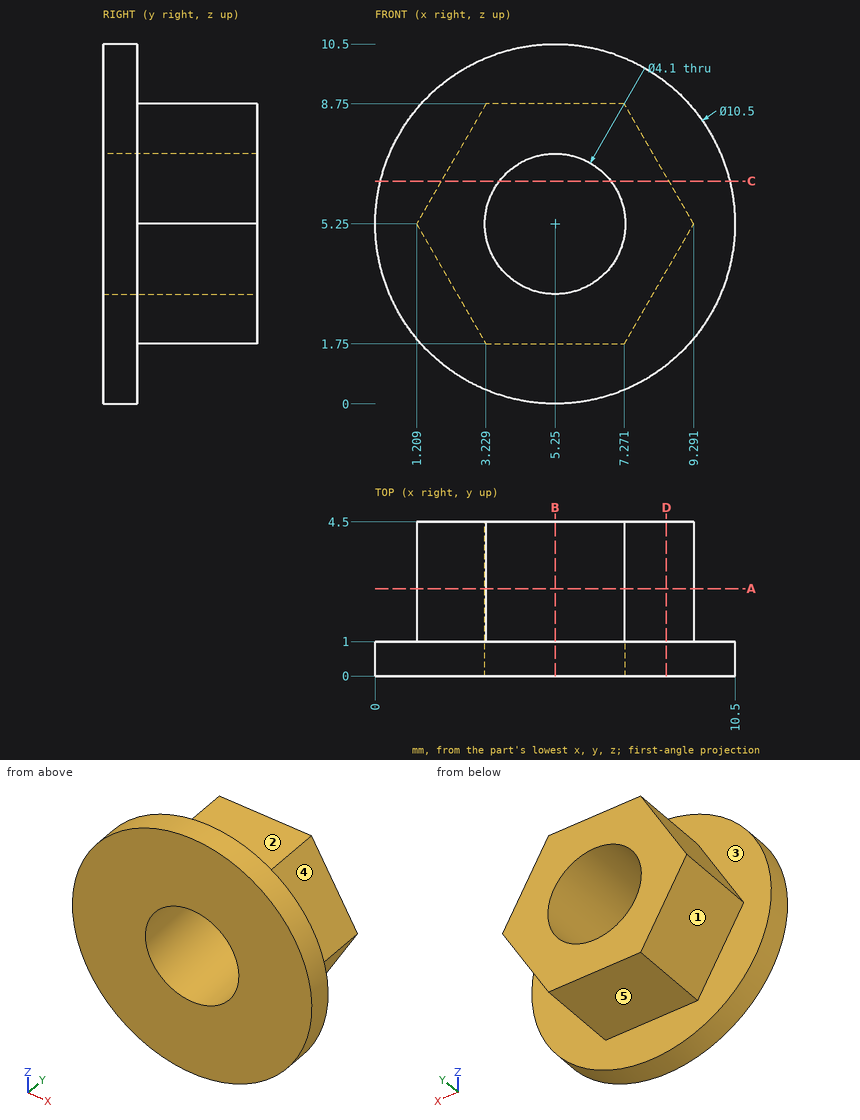
Here's the drawing with two shaded views (mm, measured from the low corner). I have some questions. A direction names the side the tool comes from. Give positions to 0.01 mm unless a question says otherwise; leave off trailing zeros. Loops run counter-clockwise (first coordinate to the right, second up) from the corner with the lowest first, then second, coordinate; pieces in that order, holes last. Notation, with made-up numbers: M 67,43 L 78,43 A12 ccw 78,58 Z; hole C 83.5,21 d5. An arc over 180 degrees is marked long. One line per item, written item: value. Start each with the question number.
1) If I drill on line 1 (Y direction, x = 0.5, z = 4.75); line 2 (X direction, y = 0.2, z = 6) (1 decimal); line 3 (X direction, y = 4, z = 5) (1 decimal), over which ranges is the centre line in solid material (lowest first)? Write a range as [from, to].
2) I'm going to push flat-ended pins straight in: pin 1 (1 mm diameter, centred on y = 2.5, z = 4.5, fed in from +X); pin 2 (1.5 mm diameter, centred on y = 3.5, z = 8, fed in from +X); pin 3 (1 mm diameter, centred on x = 5.5, y = 4, fed in from +Z). Where does each tip first touch, or does it pass through?
3) On a 3-axis mill with a long thin cutter (end or side, diameter ignored), from which of +Z, -Z, +X, -X, +Y, -Y can I reach the whole of each face in a straight line? I mean the marked faces 1, 2, 3, 4 and 5. Say none if no direction works.
4) If we section it at B-B, the plane x = 5.25: Write out the boundary of the cut face in (y, z).
5) If we section it at C-C, the plane z = 6.5: Write out the boundary of the cut face in (x, y) (1 decimal), and give its area (3 significant figures).
6) If we section it at D-D, the plane x = 8.5: Write out the boundary of the cut face in (y, z).
7) If we section it at A-A, the plane y = 2.55: Write out the boundary of the cut face in (x, z).
Completed:
1. line 1: y = [0, 1]
1. line 2: x = [0.1, 3.3], [7.2, 10.4]
1. line 3: x = [1.4, 3.2], [7.3, 9.1]
2. pin 1: stops at x = 9.15
2. pin 2: stops at x = 8.14
2. pin 3: stops at z = 8.75
3. face 1: -Z, -X, +Y
3. face 2: +Z, +X, -X, +Y
3. face 3: +Y
3. face 4: +Z, +X, +Y
3. face 5: -Z, +X, -X, +Y
4. outline: M 0,0 L 1,0 L 1,1.75 L 4.5,1.75 L 4.5,3.2 L 0,3.2 Z; M 0,7.3 L 4.5,7.3 L 4.5,8.75 L 1,8.75 L 1,10.5 L 0,10.5 Z
5. outline: M 0.2,0 L 3.6,0 L 3.6,4.5 L 1.9,4.5 L 1.9,1 L 0.2,1 Z; M 6.9,0 L 10.3,0 L 10.3,1 L 8.6,1 L 8.6,4.5 L 6.9,4.5 Z
5. area: 18.8 mm^2
6. outline: M 0,1.13 L 1,1.13 L 1,3.88 L 4.5,3.88 L 4.5,6.62 L 1,6.62 L 1,9.37 L 0,9.37 Z
7. outline: M 1.21,5.25 L 3.23,1.75 L 7.27,1.75 L 9.29,5.25 L 7.27,8.75 L 3.23,8.75 Z; hole C 5.25,5.25 d4.1
